from build123d import *

# Parameters (mm, degrees)
SKETCH1_W           = 144
SKETCH1_H           = 23
BOSS_EXTRUDE1_DEPTH = 3
FILLET1_R           = 2
BOSS_EXTRUDE2_DEPTH = 3


with BuildPart() as part:
    # Sketch1 → Boss-Extrude1 (new body)
    with BuildSketch(Plane(origin=(0, 0, 0), x_dir=(0, 0, -1), z_dir=(1, 0, 0))):
        Rectangle(SKETCH1_W, SKETCH1_H)
    extrude(amount=BOSS_EXTRUDE1_DEPTH)

    # Fillet1
    fillet1_edges = [part.edges().sort_by_distance(p)[0] for p in [
        (1.5, 11.5, 72),
        (1.5, 11.5, -72),
    ]]
    fillet(fillet1_edges, radius=FILLET1_R)

    # Sketch2 → Boss-Extrude2 (add)
    with BuildSketch(Plane(origin=(3, 0, 0), x_dir=(0, 0, -1), z_dir=(1, 0, 0))):
        Polygon((-72, -11.5), (-72, -21.5), (-42, -11.5), align=None)
        Polygon((72, -11.5), (72, -21.5), (42, -11.5), align=None)
    extrude(amount=-BOSS_EXTRUDE2_DEPTH)


solid = part.part
Input: part model. Units: mm. Frame: model coordinates. A direction names the side the tool comes from. Give positions to 0.01 mm unless a question says otherwise; leave off trailing zeros. Order: outer loops, then holes, each group sorted by start corner. A loop starts at its lowest first (then second) coordinate and runs counter-clockwise, first axis right, second up. Notation, with made-up numbers: (49, 2.5) - (59, 2.5) arc R11 ccw to (59, 11.5) - close; hole circle Ø7 at (-31, 62.25). An arc over 180 degrees is marked (long way). Answer as a JSON object with one key per item and string values. Group by question number.
Q1. Cut plane D-D, the plane z = -47.5. Output: boundary loops of the cut face in (x, y), then the cut area to 3 significant figures.
Q2. Cut plane A-A, the plane y = -16.5. Output: boundary loops of the cut face in (x, z).
Q3. Cut plane C-C, the plane z = 27. Output: boundary loops of the cut face in (x, y).
Q4. Cut plane B-B, the plane x = 2.3. Output: boundary loops of the cut face in (y, z), then the cut area to 3 significant figures.
Q5. Set-up query: faces 1 (the face through (1.52, -16.57, -57.21)), 2 (the face through (1, 11.5, 1)). Return all of +Z, -Z, +X, -X, +Y, -Y with unobstructed straight access to the full face (end or side cutting, diameter ignored); none if empty.
Q6. Mould query, pull axis Z, two halves, no side actions, for faces 3 (the face through (1, -11.5, 1)), 4 (the face through (3, -1, 1)), 5 (the face through (1, -6, -72)). Classes: pulls with the +Z half, pulls with the -Z half, needs draft (parallel to the pull), parting line crosses it, or undercut.
Q7. Line query: probe 1 along Y at (x, z) = (0.25, 25.5); probe 2 along Y at (x, z) = (0.6, -57.5); probe 3 along Z at (x, y) = (2.6, 10.5). Output: solid intervals per line, ascending.
Results:
{
 "1": {"outline": "(0, -13.33) - (3, -13.33) - (3, 11.5) - (0, 11.5) - close", "area": "74.5 mm^2"},
 "2": {"outline": "(0, -72) - (3, -72) - (3, -57) - (0, -57) - close; (0, 57) - (3, 57) - (3, 72) - (0, 72) - close"},
 "3": {"outline": "(0, -11.5) - (3, -11.5) - (3, 11.5) - (0, 11.5) - close"},
 "4": {"outline": "(-21.5, -72) - (9.5, -72) arc R2 ccw to (11.5, -70) - (11.5, 70) arc R2 ccw to (9.5, 72) - (-21.5, 72) - (-11.5, 42) - (-11.5, -42) - close", "area": "3,610 mm^2"},
 "5": {"face 1": "+X, -X, -Y", "face 2": "+Z, -Z, +X, -X, +Y"},
 "6": {"face 3": "undercut", "face 4": "needs draft", "face 5": "pulls with the -Z half"},
 "7": {"probe 1": "-11.5 to 11.5", "probe 2": "-16.67 to 11.5", "probe 3": "-71.73 to 71.73"}
}
